```python
from build123d import *

# Parameters (mm, degrees)
SKETCH1_R           = 32.15
BOSS_EXTRUDE1_DEPTH = 5.3
SKETCH2_R           = 34.75
BOSS_EXTRUDE2_DEPTH = 9.9
SKETCH3_R           = 17.8
BOSS_EXTRUDE3_DEPTH = 22.85
SKETCH4_R           = 6.325
CUT_EXTRUDE1_DEPTH  = 25.4
FILLET1_R           = 5.5
CHAMFER2_SIZE       = 1


with BuildPart() as part:
    # Sketch1 → Boss-Extrude1 (new body)
    with BuildSketch(Plane(origin=(0, 0, 0), x_dir=(1, 0, 0), z_dir=(0, 1, 0))):
        with Locations(Location((0, 0, 0), (0, 0, 270))):
            Circle(SKETCH1_R)
    extrude(amount=BOSS_EXTRUDE1_DEPTH)

    # Sketch2 → Boss-Extrude2 (add)
    with BuildSketch(Plane(origin=(0, 5.3, 0), x_dir=(1, 0, 0), z_dir=(0, 1, 0))):
        with Locations(Location((0, 0, 0), (0, 0, 90))):
            Circle(SKETCH2_R)
    extrude(amount=BOSS_EXTRUDE2_DEPTH)

    # Sketch3 → Boss-Extrude3 (add)
    with BuildSketch(Plane(origin=(0, 15.2, 0), x_dir=(1, 0, 0), z_dir=(0, 1, 0))):
        with Locations(Location((0, 0, 0), (0, 0, 90))):
            Circle(SKETCH3_R)
    extrude(amount=BOSS_EXTRUDE3_DEPTH)

    # Sketch4 → Cut-Extrude1 (cut)
    with BuildSketch(Plane(origin=(0, 38.05, 0), x_dir=(1, 0, 0), z_dir=(0, 1, 0))):
        with Locations(Location((0, 0, 0), (0, 0, 270))):
            Circle(SKETCH4_R)
    extrude(amount=-CUT_EXTRUDE1_DEPTH, mode=Mode.SUBTRACT)

    # Fillet1
    fillet1_edges = [part.edges().sort_by_distance(p)[0] for p in [
        (0, 15.2, 17.8),
    ]]
    fillet(fillet1_edges, radius=FILLET1_R)

    # Chamfer1: read off the stored shape, not the designer's step
    # Chamfer1 outline → Chamfer1 (revolve, cut)
    with BuildSketch(Plane.XY):
        Polygon((17.8, 38.05), (16.5, 38.05), (17.8, 36.75), align=None)
    revolve(axis=Axis((0, 0, 0), (0, 1, 0)), mode=Mode.SUBTRACT)

    # Chamfer2
    chamfer2_edges = [part.edges().sort_by_distance(p)[0] for p in [
        (0, 15.2, 34.75),
    ]]
    chamfer(chamfer2_edges, length=CHAMFER2_SIZE)


solid = part.part
```
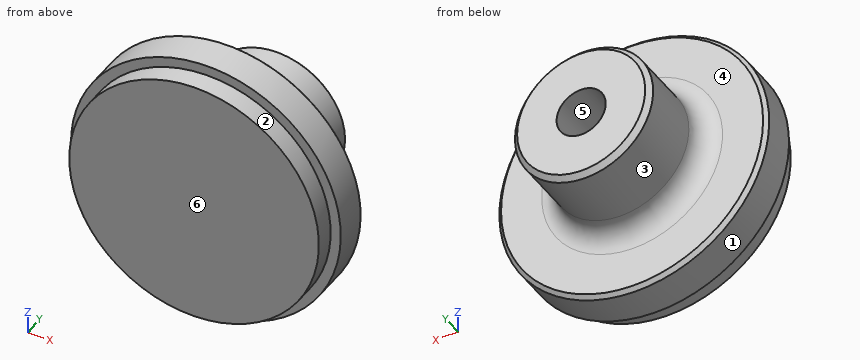
The listing builds one solid part. Answer for the finished solid, in the listing's coordinates (mm). Face numbers are marked on the shaded views. A direction names the side the tool comes from. Round coordinates to 2 decimals unless told otherwise and drop trailing zeros. Order: outer loops, then holes, each group sorted by start corner. A loop starts at its lowest first (then second) coordinate and runs counter-clockwise, first axis right, second up. Notation, with made-up numbers: (-8.5, 11) -> (45.5, 11) arc R4 cw to (45.5, 16) -> close; hole circle Ø8 at (27.25, 66.25). An arc over 180 degrees is marked (long way). Answer as CSV lines item,"result".
Q1. Consider line 1 (X direction, y = 30, z = 0) (3 decimals); line 2 (Y direction, x = -24, z = 18); line 3 (Y direction, x = -27, z = -18.5). Determine where each line is inside the solid, lowest interval first. Write a range as from..to.
Computed values:
line 1,"x = -17.8..-6.325, 6.325..17.8"
line 2,"y = 0..15.2"
line 3,"y = 5.3..15.2"
Q2. For a pull along Y with two mould halves and no side action, classify the marked faces 4, 5 and 6 as +Y half, -Y half, draft (parallel to the pull), parting line (faces both ways), or undercut.
Computed values:
face 4,"+Y half"
face 5,"draft"
face 6,"-Y half"
Q3. A cutting plane is placed at A-A on x = 0. Determine the outline of the cut face in (y, z) (3 decimals), plus the area to 3 significant figures.
Computed values:
outline,"(0, -32.15) -> (5.3, -32.15) -> (5.3, -34.75) -> (14.2, -34.75) -> (15.2, -33.75) -> (15.2, -23.3) arc R5.5 cw to (20.7, -17.8) -> (36.75, -17.8) -> (38.05, -16.5) -> (38.05, -6.325) -> (12.65, -6.325) -> (12.65, 6.325) -> (38.05, 6.325) -> (38.05, 16.5) -> (36.75, 17.8) -> (20.7, 17.8) arc R5.5 cw to (15.2, 23.3) -> (15.2, 33.75) -> (14.2, 34.75) -> (5.3, 34.75) -> (5.3, 32.15) -> (0, 32.15) -> close"
area,"1,530 mm^2"
Q4. Which of the six approach directions +Z, -Z, +X, -X, +Y, -Y give full straight-line access (tool end or side, diameter ignored) to the marked faces 1, 2 and 3?
Computed values:
face 1,"+Y, -Y"
face 2,"-Y"
face 3,"+Y"
Q5. A cutting plane is placed at D-D on y = 4. Determine the outline of the cut face in (x, z), plus the area to 3 significant figures.
Computed values:
outline,"circle Ø64.3 at (0, 0)"
area,"3,250 mm^2"
Q6. A cutting plane is placed at B-B on z = 0. Determine the outline of the cut face in (x, y) (3 decimals), plus the area to 3 significant figures.
Computed values:
outline,"(-34.75, 5.3) -> (-32.15, 5.3) -> (-32.15, 0) -> (32.15, 0) -> (32.15, 5.3) -> (34.75, 5.3) -> (34.75, 14.2) -> (33.75, 15.2) -> (23.3, 15.2) arc R5.5 cw to (17.8, 20.7) -> (17.8, 36.75) -> (16.5, 38.05) -> (6.325, 38.05) -> (6.325, 12.65) -> (-6.325, 12.65) -> (-6.325, 38.05) -> (-16.5, 38.05) -> (-17.8, 36.75) -> (-17.8, 20.7) arc R5.5 cw to (-23.3, 15.2) -> (-33.75, 15.2) -> (-34.75, 14.2) -> close"
area,"1,530 mm^2"
Q7. Given pin 1 (5 mm diameter, centred on y = 23.5, z = 4.5, fed in from +X); pin 2 (10 mm diameter, centred on y = 30.5, z = -24, fed in from -X); pin 3 (6 mm diameter, centred on x = 6.5, y = 32.5, fed in from +Z); pin 4 (12 mm diameter, centred on x = -26, y = 6.5, fed in from -Z), each flat-ended and moving along its own axis, determine where each tip first touches the part or whether it passes through.
Computed values:
pin 1,"stops at x = 17.69"
pin 2,"passes through"
pin 3,"stops at z = 17.45"
pin 4,"stops at z = -28.42"
Q8. A cutting plane is placed at C-C on y = 33. Determine the outline of the cut face in (x, z) (3 decimals), plus the area to 3 significant figures.
Computed values:
outline,"circle Ø35.6 at (0, 0); hole circle Ø12.65 at (0, 0)"
area,"870 mm^2"
